```python
from build123d import *

# Parameters (mm, degrees)
BOSS_EXTRUDE1_DEPTH     = 10
CUT_EXTRUDE4_DEPTH      = 186.673146884
CUT_EXTRUDE4_DEPTH_BACK = 186.673146884
SKETCH2_R               = 5
SKETCH3_R               = 7
CUT_EXTRUDE5_DEPTH      = 186.673146884


with BuildPart() as part:
    # Sketch1 → Boss-Extrude1 (new body)
    with BuildSketch(Plane(origin=(0, 0, 0), x_dir=(1, 0, 0), z_dir=(0, 1, 0))):
        with BuildLine():
            Line((-1.545174458, 127), (10, 127))
            ThreePointArc((10, 127), (62.706174301, 110.445628071), (96.481761872, 66.728380632))
            ThreePointArc((96.481761872, 66.728380632), (96.94422721, 65.024977681), (97.1, 63.266799465))
            Line((97.1, 63.266799465), (97.1, 10))
            ThreePointArc((97.1, 10), (94.171067812, 2.928932188), (87.1, 0))
            Line((87.1, 0), (5, 0))
            ThreePointArc((5, 0), (-2.071067812, -2.928932188), (-5, -10))
            Line((-5, -10), (-5, -30))
            ThreePointArc((-5, -30), (-7.928932188, -37.071067812), (-15, -40))
            Line((-15, -40), (-125, -40))
            ThreePointArc((-125, -40), (-132.071067812, -37.071067812), (-135, -30))
            Line((-135, -30), (-135, 20.135444575))
            ThreePointArc((-135, 20.135444575), (-134.306211211, 23.795285131), (-132.321113421, 26.947294417))
            Line((-132.321113421, 26.947294417), (-42.119413536, 123.892601626))
            ThreePointArc((-42.119413536, 123.892601626), (-38.77974787, 126.253977703), (-34.774007346, 127.080722276))
            Line((-34.774007346, 127.080722276), (-1.545174458, 127))
        make_face()
    extrude(amount=BOSS_EXTRUDE1_DEPTH)

    # Sketch2 → Cut-Extrude4 (cut, two sides: drawn at the far end of the back side and taken through both)
    with BuildSketch(Plane(origin=(0, 0, 0), x_dir=(1, 0, 0), z_dir=(0, 1, 0)).offset(-CUT_EXTRUDE4_DEPTH_BACK)):
        with Locations(Location((14.998992834, 111.984631039, 0), (0, 0, 270))):
            Circle(SKETCH2_R)
        with Locations(Location((82.1, 65, 0), (0, 0, 270))):
            Circle(SKETCH2_R)
        with Locations(Location((32.1, 65, 0), (0, 0, 270))):
            Circle(SKETCH2_R)
    extrude(amount=CUT_EXTRUDE4_DEPTH + CUT_EXTRUDE4_DEPTH_BACK, mode=Mode.SUBTRACT)

    # Sketch3 → Cut-Extrude5 (cut, through all)
    with BuildSketch(Plane.XZ):
        with Locations(Location((-70, 20, 0), (0, 0, 270))):
            Circle(SKETCH3_R)
    extrude(amount=-CUT_EXTRUDE5_DEPTH, mode=Mode.SUBTRACT)


solid = part.part
```
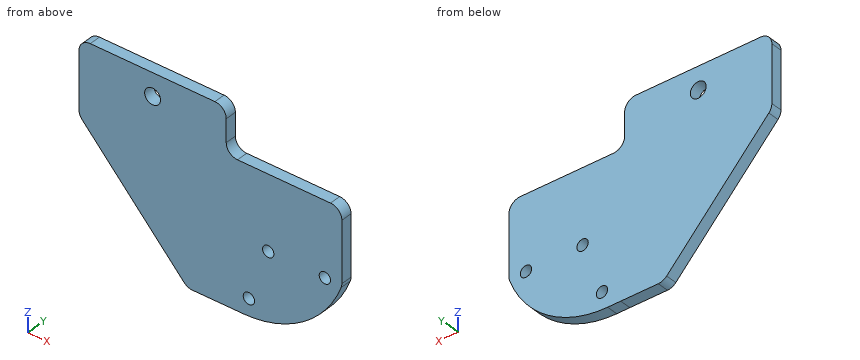
Source: CAD feature listing. Evaluate the final solid. Frame: model axes, mm. Give positions to 0.01 mm unless a question says otherwise; leave off trailing zeros. Loops run counter-clockwise (first coordinate to the right, second up) from the corner with the lowest first, then second, coordinate; pieces in that order, holes last. Notation, with made-up numbers: (42.5, -31.75) -> (88.5, -31.75) arc R29 ccw to (88.5, 7.25) -> close; hole circle Ø11 at (-13.5, -29). An arc over 180 degrees is marked (long way). Use a Markdown table: item, result. Add a question column.
(1) Ray query, line 1 (X direction, y = 6.5, z = 20); line 2 (X direction, y = 3.25, z = -65); line 3 (X direction, y = 7.5, z = 11). Return the intervals inside material, ascending.
(2) Section query C-C (x = 32.1). Output: boundary loops of the cut face in (y, z).
(3) Section query B-B (y = 6.5). Output: boundary loops of the cut face in (x, z).
(4) First-contact query: pin 1 Ø3 at (x, y) = (3.5, 3.5) entering from -Z; pin 2 Ø4 at (x, y) = (49.5, 8.5) entering from +Z; pin 3 Ø6 at (x, y) = (42.5, 2.5) entering from -Z. Flat tips, straight axial feed; report the tip coordinate or a pass-through.
(5) Section query A-A (z = 20). Output: boundary loops of the cut face in (x, y), then the cut area to 3 significant figures.
(6) Section query D-D (x = -47.5). Output: boundary loops of the cut face in (y, z).
Checked values:
| question | item | result |
|---|---|---|
| 1 | line 1 | -135 to -77, -63 to -5 |
| 1 | line 2 | -96.92 to 27.1, 37.1 to 77.1, 87.1 to 96.95 |
| 1 | line 3 | -135 to -5 |
| 2 | outline | (0, -124.31) -> (10, -124.31) -> (10, -70) -> (0, -70) -> close; (0, -60) -> (10, -60) -> (10, 0) -> (0, 0) -> close |
| 3 | outline | (-135, -20.14) arc R10 ccw to (-132.32, -26.95) -> (-42.12, -123.89) arc R10 ccw to (-34.77, -127.08) -> (-1.55, -127) -> (10, -127) arc R92.18 ccw to (96.48, -66.73) arc R10 ccw to (97.1, -63.27) -> (97.1, -10) arc R10 ccw to (87.1, 0) -> (5, 0) arc R10 cw to (-5, 10) -> (-5, 30) arc R10 ccw to (-15, 40) -> (-125, 40) arc R10 ccw to (-135, 30) -> close; hole circle Ø14 at (-70, 20); hole circle Ø10 at (15, -111.98); hole circle Ø10 at (32.1, -65); hole circle Ø10 at (82.1, -65) |
| 4 | pin 1 | z = -127 |
| 4 | pin 2 | z = 0 |
| 4 | pin 3 | z = -122.15 |
| 5 | outline | (-135, 0) -> (-77, 0) -> (-77, 10) -> (-135, 10) -> close; (-63, 0) -> (-5, 0) -> (-5, 10) -> (-63, 10) -> close |
| 5 | area | 1,160 mm^2 |
| 6 | outline | (0, -118.11) -> (10, -118.11) -> (10, 40) -> (0, 40) -> close |
